Design review of the part built by this model. Coordinates are the model's own, in mm. Face numbers are marked on the shaded views. A direction names the side the tool comes from. Give positions to 0.01 mm unless a question says otherwise; leave off trailing zeros. Write each loop counter-clockwise with the first axis right and the second up, starting at its lowest first coordinate (ties: lowest second). Pieces come first, ordered by that corner, then holes. Notation, with made-up numbers: M 48,22 L 85,22 A27 cw 85,55 Z; hole C 57,-22.5 d11. An arc over 180 degrees is marked long. Answer in a Markdown table with one row per item.
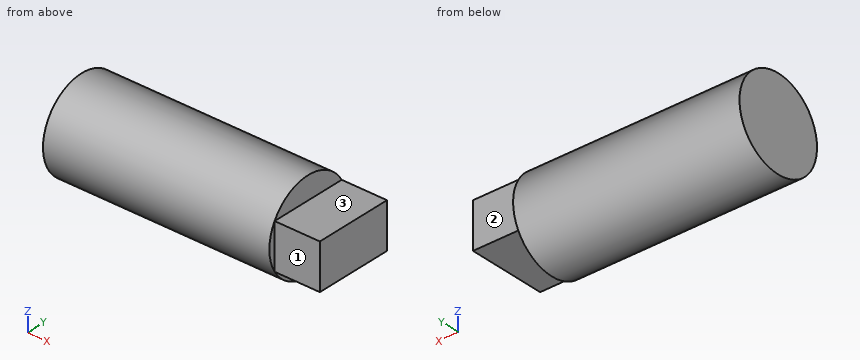
```python
from build123d import *

# Parameters (mm, degrees)
SKETCH_1_R          = 30
EXTRUDE_1_DEPTH     = 10
CUT_EXTRUDE_START   = -10
SKETCH_2_R          = 30
SKETCH_2_R_2        = 10
CUT_EXTRUDE_1_DEPTH = 10
SKETCH_4_R          = 10
EXTRUDE_2_DEPTH     = 40
SKETCH_5_W          = 10
SKETCH_5_H          = 17.320508076
EXTRUDE_3_DEPTH     = 10


with BuildPart() as part:
    # 草图1 → 凸台-拉伸1 (new body)
    with BuildSketch(Plane(origin=(0, 0, 0), x_dir=(0, 0, -1), z_dir=(1, 0, 0))):
        Circle(SKETCH_1_R)
    extrude(amount=EXTRUDE_1_DEPTH)

    # 草图2 → 切除-拉伸1 (cut)
    with BuildSketch(Plane(origin=(10, 0, 0), x_dir=(0, 0, -1), z_dir=(1, 0, 0)).offset(CUT_EXTRUDE_START)):
        Circle(SKETCH_2_R)
        Circle(SKETCH_2_R_2, mode=Mode.SUBTRACT)
    extrude(amount=CUT_EXTRUDE_1_DEPTH, mode=Mode.SUBTRACT)

    # 草图4 → 凸台-拉伸2 (add)
    with BuildSketch(Plane(origin=(10, 0, 0), x_dir=(0, 0, -1), z_dir=(1, 0, 0))):
        Circle(SKETCH_4_R)
    extrude(amount=EXTRUDE_2_DEPTH)

    # 草图5 → 凸台-拉伸3 (add)
    with BuildSketch(Plane(origin=(50, 0, 0), x_dir=(0, 0, -1), z_dir=(1, 0, 0))):
        Rectangle(SKETCH_5_W, SKETCH_5_H)
    extrude(amount=EXTRUDE_3_DEPTH)


solid = part.part
```
1) Add section D-D (z = 8). Write out the cut boundary in (x, y), and give its area (3 significant figures).
Geometry says:
| item | result |
|---|---|
| outline | M 0,-6 L 50,-6 L 50,6 L 0,6 Z |
| area | 600 mm^2 |
2) Insertion check: P1, Ø1.5, axis at y = 0.5, z = -7.5, coming from the +X side; P2, Ø8, axis at x = 7.5, z = 5.5, coming from the -Y side; P3, Ø8, axis at x = 56.5, y = -2, coming from the +Z side. Each pin has a flat end and moves straight along its axis. Give the tip position at first contact, or say it passes through.
Geometry says:
| item | result |
|---|---|
| P1 | x = 50 |
| P2 | y = -9.89 |
| P3 | z = 5 |
3) Add section B-B (y = 0). Write out the cut boundary in (x, z).
Geometry says:
| item | result |
|---|---|
| outline | M 0,-10 L 50,-10 L 50,-5 L 60,-5 L 60,5 L 50,5 L 50,10 L 0,10 Z |
4) Add section C-C (x = 56). Write out the cut boundary in (y, z), and give its area (3 significant figures).
Geometry says:
| item | result |
|---|---|
| outline | M -8.66,-5 L 8.66,-5 L 8.66,5 L -8.66,5 Z |
| area | 173 mm^2 |
5) Add section A-A (z = 0). Write out the cut boundary in (x, y).
Geometry says:
| item | result |
|---|---|
| outline | M 0,-10 L 50,-10 L 50,-8.66 L 60,-8.66 L 60,8.66 L 50,8.66 L 50,10 L 0,10 Z |
6) To check wall thickness, follow probe 1 along Y at (x, z) = (4.5, 5); probe 2 along X at (y, z) = (-1.25, -5.25); probe 3 along Z at (x, y) = (53.5, 4.25). State the ranges of each line that lie inside material, in increasing order. Write a range as [from, to].
Geometry says:
| item | result |
|---|---|
| probe 1 | [-8.66, 8.66] |
| probe 2 | [0, 50] |
| probe 3 | [-5, 5] |
7) For the marked faces 1, 2 and 3, list the 3-axis set-ups (+Z, -Z, +X, -X, +Y, -Y) from which the entire face can be reached by the end or side of a thin tool; tool diameter is ignored.
Geometry says:
| item | result |
|---|---|
| face 1 | +Z, -Z, +X, -Y |
| face 2 | +Z, -Z, +X, +Y |
| face 3 | +Z, +X, +Y, -Y |
